Autodesk Fusion 360 part; units mm, degrees
sketch "Skizze1" plane through (0, 0, 0) normal (0, 0, 1) x (1, 0, 0)
  circle A0 centre (0, 0) radius 1.8
  circle A1 centre (-28, 0) radius 1.8
  line L0 (-28, 0) -> (0, 0) construction
  line L1 (-28, 3) -> (0, 3)
  line L2 (-28, -3) -> (0, -3)
  arc A2 (-28, 3) -> (-28, -3) centre (-28, 0) ccw
  arc A3 (0, -3) -> (0, 3) centre (0, 0) ccw
  dimension "d1" = 3.6
  dimension "d2" = 28
  dimension "d3" = 6
extrude "Extrusion1" add sketch "Skizze1" along normal blind 3
sketch "Skizze2" plane through (0, 0, 0) normal (0, 0, 1) x (-1, 0, 0)
  circle A0 centre (0, 0) radius 1.8
  circle A1 centre (28, 0) radius 1.8
  arc A2 (28, -3) -> (28, 3) centre (28, 0) ccw
  line L0 (28, 3) -> (0, 3)
  arc A3 (0, 3) -> (0, -3) centre (0, 0) ccw
  line L1 (0, -3) -> (28, -3)
  line L2 (24.75, -3) -> (3.25, -3)
  line L3 (3.25, -3) -> (3.25, 3.7)
  line L4 (3.25, 3.7) -> (24.75, 3.7)
  line L5 (24.75, 3.7) -> (24.75, -3)
  circle A4 centre (0, 0) radius 1.8
  circle A5 centre (28, 0) radius 1.8
  arc A6 (28, -3) -> (28, 3) centre (28, 0) ccw
  line L6 (28, -3) -> (0, -3)
  arc A7 (0, 3) -> (0, -3) centre (0, 0) ccw
  line L7 (0, 3) -> (28, 3)
  line L8 (28, 0) -> (0, 0) construction
  line L9 (14, 0) -> (14, 18.5057) construction
  dimension "d9" = 0.7
  dimension "d10" = 21.5
extrude "Extrusion2" add sketch "Skizze2" against normal blind 8.23 contours L0 L1 L2 L3 L5 L6 L7 | L0 L3 L4 L5 L7
sketch "Skizze3" plane through (0, 3, 0) normal (0, 1, 0) x (-1, 0, 0)
  line L0 (24.75, 0) -> (28, 0)
  line L1 (28, 0) -> (28, 3)
  line L2 (28, 3) -> (0, 3)
  line L3 (0, 3) -> (0, 0)
  line L4 (0, 0) -> (3.25, 0)
  line L5 (3.25, 0) -> (3.25, -8.23)
  line L6 (3.25, -8.23) -> (24.75, -8.23)
  line L7 (24.75, -8.23) -> (24.75, 0)
  circle A0 centre (22.25, -5.73) radius 1.05
  circle A1 centre (5.75, -5.73) radius 1.05
  line L8 (24.75, -5.73) -> (3.25, -5.73) construction
  dimension "d11" = 2.1
  dimension "d13" = 2.5
  dimension "d14" = 2.5
  dimension "d15" = 2.5
extrude "Extrusion3" cut sketch "Skizze3" against normal up to surface (6.7 mm away) contours A0 | A1
chamfer "Fase1" distance 1 angle 45 3 edges at (-24.75, 3, -4.115) (-14, 3, -8.23) (-3.25, 3, -4.115)
sketch "Skizze4" plane through (-24.75, 0, 0) normal (-1, 0, 0) x (0, -1, 0)
  line L0 (-2, 0) -> (-2, -8.23)
  line L1 (-2, -8.23) -> (3.7, -8.23)
  line L2 (3.7, -8.23) -> (3.7, 0)
  line L3 (3.7, 0) -> (3, 0)
  line L4 (3, 0) -> (-2, 0)
  line L5 (3.7, -4.68) -> (3.7, -6.78)
  line L6 (3.7, -4.68) -> (3.7, -6.78)
  line L7 (3.7, 0) -> (3.7, -8.23)
  line L8 (3.7, -8.23) -> (3.7, 0)
  line L9 (3, 0) -> (3, 3)
  line L10 (3, 3) -> (3, 0)
  line L11 (3, 0) -> (3.7, 0)
  line L12 (3.7, 0) -> (3, 0)
  line L13 (3.7, -3.23) -> (3.7, 0)
  line L14 (3, 0) -> (3.7, -3.23)
  dimension "d29" = 5
extrude "Extrusion4" cut sketch "Skizze4" against normal up to surface (21.5 mm away) contours L2 L3 L7 L8 L11 L12 L13 L14
sketch "Skizze5" plane through (0, 0, -8.23) normal (0, 0, -1) x (1, 0, 0)
  line L0 (-24.75, -2) -> (-3.25, -2)
  line L1 (-3.25, -2) -> (-3.25, 3.7)
  line L2 (-3.25, 3.7) -> (-24.75, 3.7)
  line L3 (-24.75, 3.7) -> (-24.75, -2)
  line L4 (-19.75, 3.7) -> (-16.8937, 1.7)
  line L5 (-16.8937, 1.7) -> (-11.1063, 1.7)
  line L6 (-11.1063, 1.7) -> (-8.25, 3.7)
  line L7 (-14, 3.7) -> (-14, -2) construction
  line L8 (-19.75, 3.7) -> (-8.25, 3.7)
  dimension "d22" = 5
  dimension "d24" = 2
  dimension "d25" = 35
extrude "Extrusion5" cut sketch "Skizze5" against normal up to surface (11.23 mm away) contours L2 L4 L5 L6 L8
equation "d7 = -6.73 mm - 1.5 mm"
equation "d13 = 1 mm + 1.5 mm"
equation "d14 = 1 mm + 1.5 mm"
equation "d15 = 1 mm + 1.5 mm"
equation "d22 = 1 mm + 3 mm + 1 mm"
equation "d29 = 1 mm + 3 mm + 1 mm"
Build history of the part. All positions in model axes, mm. A direction names the side the tool comes from. Round coordinates to 2 decimals unless told otherwise and drop trailing zeros. Loops run counter-clockwise (first coordinate to the right, second up) from the corner with the lowest first, then second, coordinate; pieces in that order, holes last. Notation, with made-up numbers: (32, -19.5) -> (59, -19.5) arc R23 ccw to (59, 14.5) -> close; hole circle Ø7 at (69.5, 11.25). An arc over 180 degrees is marked (long way). One line per item, written item: value. Start each with the question number.
Q1. 3-axis set-ups, long thin cutter, end or side, ignore diameter. For faces 1 (the face through (-3.25, -1, -4)), 2 (the face through (-24.75, -1, -4)), 3 (the face through (-24.26, 2.49, -4.17)): which of +Z, -Z, +X, -X, +Y, -Y reach the whole face in a straight line?
Q2. Cut at D-D on x = -12.5. List the corners of the cut face in (y, z).
Q3. Probe line 1 along Y through (x, z) = (0, 1.7); line 2 along Z through (x, y) = (-5.75, -1.5); line 3 along X through (y, z) = (-0.75, -5.25). List the from-to ranges inside material, lowest first.
Q4. Two-plate mould, pull along Z, no slides. Class faces 4 (the face through (-4.92, -0.3, -6.37)), 5 (the face through (-14, 3, -2)), 6 (the face through (-14, 0, 3)): released by +Z, released by -Z, zero draft, split by the parting line, or undercut.
Q5. Cut at B-B on x = -22.25. List the corners of the cut face in (y, z).
Q6. Cut at C-C on y = -2.5. List the corners of the cut face in (x, z).
Q7. Drop flat-ended pins along their axis: pin 1 Ø3.5 at (x, z) = (-22, 1) entering from -Y; pin 2 Ø3 at (x, y) = (-1.5, 1) entering from -Z; pin 3 Ø4.5 at (x, z) = (-14.5, -2.5) entering from -Y; pin 4 Ø1.7 at (x, z) = (-5.75, -5.73) entering from +Y. Give the stop position or say it passes through.
Q8. Cut at A-A on y = 0. List the corners of the cut face in (x, z).
Computed:
1. face 1: -Z, +X, +Y, -Y
1. face 2: -Z, -X, +Y, -Y
1. face 3: -Z, -X, +Y
2. outline: (-1.7, -8.23) -> (2, -8.23) -> (3, -7.23) -> (3, 3) -> (-1.7, 3) -> close
3. line 1: -3 to -1.8, 1.8 to 3
3. line 2: -8.23 to -6.78, -4.68 to 3
3. line 3: -24.75 to -23.18, -21.32 to -6.68, -4.82 to -3.25
4. face 4: undercut
4. face 5: zero draft
4. face 6: released by +Z
5. outline: (-3.7, -8.23) -> (2, -8.23) -> (3, -7.23) -> (3, -6.78) -> (-3.7, -6.78) -> close; (-3.7, -4.68) -> (3, -4.68) -> (3, 3) -> (-3, 3) -> (-3, 0) -> (-3.7, -3.23) -> close
6. outline: (-29.66, 0) -> (-24.75, 0) -> (-24.75, -8.23) -> (-18.04, -8.23) -> (-18.04, 3) -> (-29.66, 3) -> close; (-9.96, -8.23) -> (-3.25, -8.23) -> (-3.25, 0) -> (1.66, 0) -> (1.66, 3) -> (-9.96, 3) -> close; hole circle Ø2.1 at (-22.25, -5.73); hole circle Ø2.1 at (-5.75, -5.73)
7. pin 1: y = -3.16
7. pin 2: z = 0
7. pin 3: y = -1.7
7. pin 4: through
8. outline: (-31, 0) -> (-29.8, 0) -> (-29.8, 3) -> (-31, 3) -> close; (-26.2, 0) -> (-24.75, 0) -> (-24.75, -8.23) -> (-3.25, -8.23) -> (-3.25, 0) -> (-1.8, 0) -> (-1.8, 3) -> (-26.2, 3) -> close; (1.8, 0) -> (3, 0) -> (3, 3) -> (1.8, 3) -> close; hole circle Ø2.1 at (-22.25, -5.73); hole circle Ø2.1 at (-5.75, -5.73)
